Design review of the part built by this model. Coordinates are the model's own, in mm. A direction names the side the tool comes from. Give positions to 0.01 mm unless a question says otherwise; leave off trailing zeros. Write each loop counter-clockwise with the first axis right and the second up, starting at its lowest first coordinate (ties: lowest second). Pieces come first, ordered by that corner, then holes. Notation, with made-up numbers: (82.5, 11) -> (124.5, 11) arc R24 cw to (124.5, 49) -> close; hole circle Ø1 at (5.25, 21). An arc over 180 degrees is marked (long way). Answer as a JSON object with one key per item and string values.
```python
from build123d import *

# Parameters (mm, degrees)
F1_DEPTH  = 76.2
F2_W      = 6.35
F2_H      = 3.175
F2_W_2    = 11.938
F3_DEPTH  = 76.201
F5_DEPTH  = 1.778
F7_DEPTH  = 3.81
F9_DEPTH  = 6.351
F11_DEPTH = 1.27
F13_DEPTH = 5.08


with BuildPart() as f1:
    # F0 (on Front) → F1 (new body)
    with BuildSketch(Plane.XZ):
        Polygon((-15.875, 9.525), (-19.05, 0), (19.05, 0), (15.875, 9.525), align=None)
    extrude(amount=F1_DEPTH)

    # F2 (on face) → F3 (cut, through all)
    with BuildSketch(Plane.XZ.offset(76.2)):
        with Locations((10.922, 7.9375)):
            Rectangle(F2_W, F2_H)
        with Locations((0, 7.9375)):
            Rectangle(F2_W_2, F2_H)
        with Locations((-10.922, 7.9375)):
            Rectangle(F2_W, F2_H)
        Polygon((-16.002, 3.81), (-17.272, 0), (17.272, 0), (16.002, 3.81), align=None)
    extrude(amount=-F3_DEPTH, mode=Mode.SUBTRACT)

    # F4 (on face) → F5 (join)
    with BuildSketch(Plane.XZ.offset(76.2)):
        Polygon((-15.875, 9.525), (-19.05, 0), (19.05, 0), (15.875, 9.525), (14.097, 9.525), (14.097, 6.35), (7.747, 6.35), (7.747, 9.525), (5.969, 9.525), (5.969, 6.35), (-5.969, 6.35), (-5.969, 9.525), (-7.747, 9.525), (-7.747, 6.35), (-14.097, 6.35), (-14.097, 9.525), align=None)
    extrude(amount=-F5_DEPTH)

    # F6 (on face) → F7 (join, through all)
    with BuildSketch(Plane(origin=(0, 0, 3.81), x_dir=(1, 0, 0), z_dir=(0, 0, -1))):
        with BuildLine():
            Line((-8.48241, 74.422), (-13.36159, 74.422))
            ThreePointArc((-13.36159, 74.422), (-10.922, 69.215), (-8.48241, 74.422))
        make_face()
    extrude(amount=F7_DEPTH)

    # F8 (on face) → F9 (cut, through all)
    with BuildSketch(Plane.XY.offset(6.35)):
        with BuildLine():
            Line((-9.017, -76.2), (-9.017, -74.93))
            ThreePointArc((-9.017, -74.93), (-10.922, -69.215), (-12.827, -74.93))
            Line((-12.827, -74.93), (-12.827, -76.2))
            Line((-12.827, -76.2), (-9.017, -76.2))
        make_face()
    extrude(amount=-F9_DEPTH, mode=Mode.SUBTRACT)

    # F10 (on face) → F11 (join)
    with BuildSketch(Plane.XY.offset(6.35)):
        with BuildLine():
            Line((9.038063, -76.2), (9.038063, -77.036362))
            ThreePointArc((9.038063, -77.036362), (8.508657, -79.532069), (10.414, -81.228682))
            Line((10.414, -81.228682), (10.414, -78.047838))
            Line((10.414, -78.047838), (11.43, -78.047838))
            Line((11.43, -78.047838), (11.43, -81.228682))
            ThreePointArc((11.43, -81.228682), (13.335343, -79.532069), (12.805937, -77.036362))
            Line((12.805937, -77.036362), (12.805937, -76.2))
            Line((12.805937, -76.2), (9.038063, -76.2))
        make_face()
    extrude(amount=-F11_DEPTH)

    # F12 (on face) → F13 (join, through all)
    with BuildSketch(Plane(origin=(0, 0, 5.08), x_dir=(1, 0, 0), z_dir=(0, 0, -1))):
        with BuildLine():
            Line((12.805937, 76.2), (12.805937, 77.036362))
            ThreePointArc((12.805937, 77.036362), (13.335343, 79.532069), (11.43, 81.228682))
            Line((11.43, 81.228682), (11.43, 80.176841))
            ThreePointArc((11.43, 80.176841), (12.432533, 78.942152), (11.789937, 77.487298))
            Line((11.789937, 77.487298), (11.789937, 76.2))
            Line((11.789937, 76.2), (12.805937, 76.2))
        make_face()
        with BuildLine():
            ThreePointArc((10.414, 81.228682), (8.508657, 79.532069), (9.038063, 77.036362))
            Line((9.038063, 77.036362), (9.038063, 76.2))
            Line((9.038063, 76.2), (10.054063, 76.2))
            Line((10.054063, 76.2), (10.054063, 77.487298))
            ThreePointArc((10.054063, 77.487298), (9.411467, 78.942152), (10.414, 80.176841))
            Line((10.414, 80.176841), (10.414, 81.228682))
        make_face()
    extrude(amount=F13_DEPTH)


solid = f1.part
```
(1) We need section B-B, the plane z = 7.25. State the section outline as (x, y) points, then the cut area to 3 significant figures.
Here are the results:
{"outline": "(-16.63, -76.2) -> (-14.1, -76.2) -> (-14.1, 0) -> (-16.63, 0) -> close; (-7.75, -76.2) -> (-5.97, -76.2) -> (-5.97, 0) -> (-7.75, 0) -> close; (5.97, -76.2) -> (7.75, -76.2) -> (7.75, 0) -> (5.97, 0) -> close; (14.1, -76.2) -> (16.63, -76.2) -> (16.63, 0) -> (14.1, 0) -> close", "area": "658 mm²"}
(2) We need section C-C, the plane x = -4. State the section outline as (y, z) points, then the cut area to 3 significant figures.
Here are the results:
{"outline": "(-76.2, 0) -> (-74.42, 0) -> (-74.42, 3.81) -> (0, 3.81) -> (0, 6.35) -> (-76.2, 6.35) -> close", "area": "200 mm²"}
(3) For faces 1 (the flat face through (-15, -74.422, 2)), 2 (the flat face through (5.969, -39, 8)), 3 (the flat face through (10.414, -80.4, 3.9)), 4 (the cylindrical face through (9.41, -78.92, 2.58)), 5 (the flat face through (7, -38, 9.525)), list the 3-axis set-ups (+Z, -Z, +X, -X, +Y, -Y) from which the entire face can be reached by the end or side of a thin tool; tool diameter is ignored.
Here are the results:
{"face 1": "-Z, +Y", "face 2": "+Z, +Y, -Y", "face 3": "+Z, -Z, -Y", "face 4": "-Z", "face 5": "+Z, +X, -X, +Y, -Y"}
(4) We need section A-A, the plane y = -57. State the section outline as (x, z) points (3 decimals), then the cut area to 3 significant figures.
Here are the results:
{"outline": "(-19.05, 0) -> (-17.272, 0) -> (-16.002, 3.81) -> (16.002, 3.81) -> (17.272, 0) -> (19.05, 0) -> (15.875, 9.525) -> (14.097, 9.525) -> (14.097, 6.35) -> (7.747, 6.35) -> (7.747, 9.525) -> (5.969, 9.525) -> (5.969, 6.35) -> (-5.969, 6.35) -> (-5.969, 9.525) -> (-7.747, 9.525) -> (-7.747, 6.35) -> (-14.097, 6.35) -> (-14.097, 9.525) -> (-15.875, 9.525) -> close", "area": "128 mm²"}
(5) The part is to be moulded in two halves that separate along X. For faces 6 (the cylindrical face through (8.5, -79.5, 3.2)), 7 (the flat face through (-7.747, -39, 8)), 8 (the flat face through (15, -38, 9.525)), say which applies: +X half, -X half, draft (parallel to the pull), parting line (faces both ways), or undercut.
Here are the results:
{"face 6": "-X half", "face 7": "undercut", "face 8": "draft"}
(6) For line 1 along X through (y, z) = (-72.5, 7.5); line 2 along X through (y, z) = (-8.5, 8.5); line 3 along Y through (x, z) = (0, 1.75), list the stretches that pass through material, from the lowest coordinate up.
Here are the results:
{"line 1": "x = -16.55 to -14.1, -7.75 to -5.97, 5.97 to 7.75, 14.1 to 16.55", "line 2": "x = -16.22 to -14.1, -7.75 to -5.97, 5.97 to 7.75, 14.1 to 16.22", "line 3": "y = -76.2 to -74.42"}
(7) Clearance check with flat-ended pins moving along their axes: pin 1 (3 mm diameter, centred on y = -48, z = 8, fed in from -X); pin 2 (1 mm diameter, centred on y = -52, z = 8.5, fed in from -X); pin 3 (2 mm diameter, centred on x = -0.5, z = 4, fed in from -Y). State where each tip first meets the part, or that it passes through.
Here are the results:
{"pin 1": "stops at x = -16.88", "pin 2": "stops at x = -16.38", "pin 3": "stops at y = -76.2"}
